Part model, mm, in its own coordinate system. Face numbers are marked on the shaded views. Give positions to 0.01 mm unless a question says otherwise; leave off trailing zeros. Write each loop counter-clockwise with the first axis right and the second up, starting at its lowest first coordinate (ties: lowest second). Pieces come first, ordered by that corner, then holes.
from build123d import *

# Parameters (mm, degrees)
F0_R     = 106.5
F0_R_2   = 75
F0_R_3   = 13.5
F0_R_4   = 37.5
F1_DEPTH = 30


with BuildPart() as f1:
    # F0 (on Front) → F1 (new body)
    with BuildSketch(Plane.XZ):
        with Locations((-61.070058, 14.18888)):
            Circle(F0_R)
        with Locations((-61.070058, 14.18888)):
            Circle(F0_R_2, mode=Mode.SUBTRACT)
        with Locations((-61.070058, 14.18888)):
            Circle(F0_R_2)
        with Locations((-115.501099, 0)):
            Circle(F0_R_3, mode=Mode.SUBTRACT)
        with Locations((-94.352807, -31.157798)):
            Circle(F0_R_3, mode=Mode.SUBTRACT)
        with Locations((-61.070058, -42.06112)):
            Circle(F0_R_3, mode=Mode.SUBTRACT)
        with Locations((-20.591359, -24.869249)):
            Circle(F0_R_3, mode=Mode.SUBTRACT)
        with Locations((-6.639018, 0)):
            Circle(F0_R_3, mode=Mode.SUBTRACT)
        with Locations((-114.308244, 32.348122)):
            Circle(F0_R_3, mode=Mode.SUBTRACT)
        with Locations((-91.748219, 61.336658)):
            Circle(F0_R_3, mode=Mode.SUBTRACT)
        with Locations((-61.070058, 14.18888)):
            Circle(F0_R_4, mode=Mode.SUBTRACT)
        with Locations((-20.883485, 53.547511)):
            Circle(F0_R_3, mode=Mode.SUBTRACT)
        with Locations((-61.070058, 70.43888)):
            Circle(F0_R_3, mode=Mode.SUBTRACT)
    extrude(amount=F1_DEPTH)


solid = f1.part
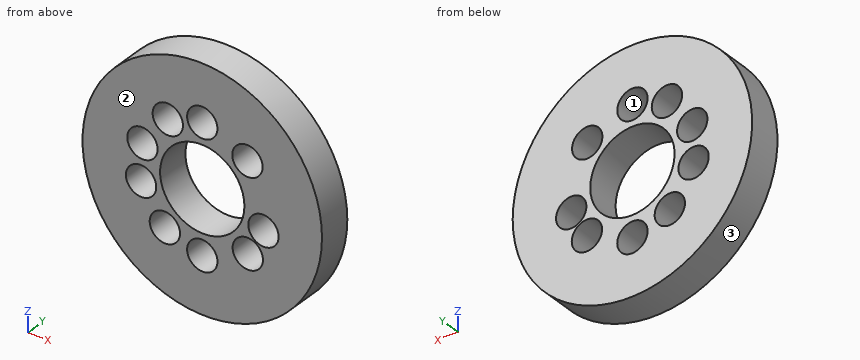
1) Saw through at B-B (y = -26.5). State how many separate pieces and enclosed holes the cut face has, and give its area (3 significant figures).
Check result:
separate pieces: 1
enclosed holes: 10
area: 26,100 mm2
2) Mould opens along X. For the marked faces 1, 2 and 3 say: +X half, -X half, draft (parallel to the pull), parting line (faces both ways), or undercut.
Check result:
face 1: undercut
face 2: draft
face 3: parting line
3) Saw through at A-A (z = -35). Write the cut outline in (x, y), and give its area (3 significant figures).
Check result:
outline: (-155.53, -30) - (-107.29, -30) - (-107.29, 0) - (-155.53, 0) - close; (-81.41, -30) - (-72.58, -30) - (-72.58, 0) - (-81.41, 0) - close; (-49.56, -30) - (-29.51, -30) - (-29.51, 0) - (-49.56, 0) - close; (-11.67, -30) - (33.39, -30) - (33.39, 0) - (-11.67, 0) - close
area: 3,670 mm2
4) Saw through at D-D (x = -154.5). Write the cut outline in (y, z).
Check result:
outline: (-30, -36.93) - (0, -36.93) - (0, 65.31) - (-30, 65.31) - close
5) Flat gauge pins, fed straight in: P1, Ø1, axis at y = -26, z = -14, coming from the -X side; P2, Ø16, axis at x = -114.31, z = 32.35, coming from the -Y side; P3, Ø1, axis at x = -107, y = -14, coming from the -Z side; P4, Ø3, axis at y = -17, z = 13.5, coming from the +X side. Where does each tip first touch, or does it go through?
Check result:
P1: stops at x = -163.91
P2: passes through
P3: stops at z = -82.14
P4: stops at x = 45.43
6) Saw through at C-C (z = 28). Write the cut outline in (x, y).
Check result:
outline: (-166.67, -30) - (-127.09, -30) - (-127.09, 0) - (-166.67, 0) - close; (-101.53, -30) - (-95.93, -30) - (-95.93, 0) - (-101.53, 0) - close; (-26.21, -30) - (44.53, -30) - (44.53, 0) - (-26.21, 0) - close
7) Drill centre lines: L1, parallel to X at y = -10.5, z = -28; L2, parallel to Z at x = -83.5, y = -5.5; L3, parallel to X at y = -16, z = 71. Where is each one in solid material? Low to high.
Check result:
L1: x = -158.86 to -107.48, -81.23 to -33.72, -7.46 to 36.72
L2: z = -89.92 to -39.19, -23.13 to -15.86, 44.24 to 50.65, 72.02 to 118.3
L3: x = -151.15 to -101.18, -82.32 to -74.56, -47.58 to 29.01
